Autodesk Inventor part; units mm, degrees
ref_plane "Work Plane1" through (0, 0, -15) normal (0, 0, 1) x (1, 0, 0)
ref_plane "YZ Plane" through (0, 0, 0) normal (1, 0, 0) x (0, 1, 0)
ref_plane "XZ Plane" through (0, 0, 0) normal (0, 1, 0) x (-1, 0, 0)
sketch "Sketch1" plane through (0, 0, 0) normal (0, 0, 1) x (1, 0, 0)
  line L0 (0, 0) -> (25, 0)
  line L1 (25, 0) -> (25, 40)
  line L2 (25, 40) -> (0, 40)
  line L3 (0, 40) -> (0, 0)
  dimension "d1" = 25
  dimension "d2" = 40
  dimension "d3" = 25
extrude "Extrusion1" add sketch "Sketch1" against normal blind 30
sketch "Sketch2" plane through (25, 0, 0) normal (1, 0, 0) x (0, 0, -1)
  line L0 (0, 0) -> (30, 0)
  circle A0 centre (15, 6.56) radius 2.46
extrude "Extrusion2" cut sketch "Sketch2" against normal blind 30
sketch "Sketch3" plane through (0, 0, 0) normal (-1, 0, 0) x (0, 0, 1)
  line L0 (0, 0) -> (-30, 0)
  line L1 (-25.05, 0) -> (-4.95, 0)
  line L2 (-4.95, 0) -> (-4.95, 33.12)
  line L3 (-4.95, 33.12) -> (-25.05, 33.12)
  line L4 (-25.05, 33.12) -> (-25.05, 0)
  dimension "d11" = 20.1
extrude "Extrusion3" cut sketch "Sketch3" against normal blind 20
sketch "Sketch4" plane through (0, 0, 0) normal (0, -1, 0) x (1, 0, 0)
  line L0 (20, -4.95) -> (20, -25.05)
  line L1 (20, -15) -> (25, -15)
  line L2 (25, 0) -> (25, -30)
  line L3 (20, -8.025) -> (25, -8.025)
  line L4 (25, -8.025) -> (25, -21.975)
  line L5 (25, -21.975) -> (20, -21.975)
  line L6 (20, -21.975) -> (20, -8.025)
  line L7 (20, -8.025) -> (25, -21.975) construction
  line L8 (25, -8.025) -> (20, -21.975) construction
  line L9 (25, -12.54) -> (25, -17.46)
  point P0 (0, 0)
  point P1 (22.5, -15)
  dimension "d14" = 13.95
extrude "Extrusion4" add sketch "Sketch4" along normal blind 15
sketch "Sketch5" plane through (20, 0, 0) normal (-1, 0, 0) x (0, 0, 1)
  circle A0 centre (-15, 6.56) radius 2.46
  circle A1 centre (-15, 6.56) radius 4.7025
  circle A2 centre (-15, 6.56) radius 2.46
  circle A3 centre (-15, 6.56) radius 2.46
  point P0 (0, 0)
  dimension "d17" = 9.405
extrude "Extrusion5" cut sketch "Sketch5" against normal blind 2.1
sketch "Sketch6" plane through (25, 0, 0) normal (1, 0, 0) x (0, 0, -1)
  circle A0 centre (15, 6.56) radius 4.7025
  line L0 (15, 6.56) -> (15, 23.56)
  circle A1 centre (15, 23.56) radius 2.46
  point P0 (0, 0)
  dimension "d20" = 17
  dimension "d21" = 4.92
extrude "Extrusion6" cut sketch "Sketch6" against normal blind 10 contours A1
sketch "Sketch7" plane through (20, 0, 0) normal (-1, 0, 0) x (0, 0, 1)
  circle A0 centre (-15, 23.56) radius 2.46
  circle A1 centre (-15, 23.56) radius 4.7025
  point P0 (0, 0)
  dimension "d24" = 9.405
extrude "Extrusion7" cut sketch "Sketch7" against normal blind 2.1
sketch "Sketch9" plane through (25, 0, 0) normal (1, 0, 0) x (0, 0, -1)
  circle A0 centre (15, 6.56) radius 2.46
  circle A1 centre (15, 6.56) radius 2.46
  circle A2 centre (15, 23.56) radius 2.46
  circle A3 centre (15, 23.56) radius 2.46
  line L0 (30, 40) -> (30, 0)
  line L1 (30, 0) -> (30, 40)
  line L2 (30, 40) -> (0, 40)
  line L3 (0, 40) -> (0, 0)
  line L4 (0, 0) -> (8.025, 0)
  line L5 (21.975, 0) -> (21.975, -15)
  line L6 (21.975, -15) -> (8.025, -15)
  line L7 (8.025, -15) -> (8.025, 0)
  line L8 (0, 0) -> (8.025, 0)
  line L9 (21.975, 0) -> (30, 0)
extrude "Extrusion8" add sketch "Sketch9" along normal blind 5
sketch "Sketch10" plane through (0, 40, 0) normal (0, 1, 0) x (1, 0, 0)
  line L0 (0, 30) -> (30, 30)
  line L1 (30, 0) -> (0, 0)
  line L2 (0, 30) -> (30, 30)
  line L3 (30, 30) -> (30, 0)
  line L4 (30, 0) -> (0, 0)
  line L5 (0, 0) -> (0, 30)
extrude "Extrusion9" add sketch "Sketch10" along normal blind 30
sketch "Sketch12" plane through (30, 0, 0) normal (1, 0, 0) x (0, 0, -1)
  circle A0 centre (15, 6.56) radius 2.46
  line L0 (15, 6.56) -> (15, 15.06)
  circle A1 centre (15, 15.06) radius 2.525
  point P0 (0, 0)
  dimension "d31" = 8.5
  dimension "d33" = 5.05
extrude "Extrusion10" cut sketch "Sketch12" against normal blind 30 contours A1
sketch "Sketch14" plane through (0, 0, 0) normal (0, 0, 1) x (1, 0, 0)
  line L0 (30, 70) -> (0, 70)
  line L1 (0, 100) -> (-8, 100)
  line L2 (30, 0) -> (30, 70)
  line L3 (30, 118) -> (30, 70)
  line L4 (30, 105) -> (30, 100)
  line L5 (0, 70) -> (30, 70)
  line L6 (0, 70) -> (0, 100)
  line L7 (-8, 145) -> (15, 145)
  line L8 (-2, 142.5) -> (-8, 145)
  line L9 (-2, 102.5) -> (-8, 100)
  line L10 (-2, 102.5) -> (4, 122.5)
  line L11 (4, 122.5) -> (-2, 142.5)
  line L12 (15, 145) -> (30, 122.5)
  line L13 (30, 122.5) -> (30, 118)
  point P0 (0, 0)
  dimension "d47" = 30
  dimension "d85" = 45
extrude "Extrusion12" add sketch "Sketch14" against normal blind 30
sketch "Sketch15" plane through (0, 0, -25.05) normal (-1, 0, 0) x (0, 0, 1)
  line L0 (0, 33.12) -> (20.1, 33.12)
  line L1 (20.1, 33.12) -> (20.1, 0)
  line L2 (0, 33.12) -> (20.1, 33.12)
  line L3 (20.1, 33.12) -> (20.1, 31.1)
  line L4 (20.1, 31.1) -> (0, 31.1)
  line L5 (0, 31.1) -> (0, 33.12)
  point P0 (25.05, 0)
  dimension "d57" = 2.02
extrude "Extrusion13" add sketch "Sketch15" against normal blind 20
sketch "Sketch25" plane through (0, 0, 0) normal (0, 0, 1) x (1, 0, 0)
  line L0 (-8, 100) -> (0, 100)
  line L1 (0, 100) -> (-8, 100)
  line L2 (-8, 100) -> (-2, 102.5)
  line L3 (-8, 100) -> (-2, 102.5)
  line L4 (-2, 102.5) -> (4, 122.5)
  line L5 (-8, 145) -> (-2, 142.5)
  line L6 (4, 122.5) -> (-2, 142.5)
  line L7 (-2, 142.5) -> (-8, 145)
  line L8 (15, 145) -> (-8, 145)
  line L9 (-8, 145) -> (15, 145)
  line L10 (15, 145) -> (30, 122.5)
  line L11 (15, 145) -> (30, 122.5)
  line L12 (30, 122.5) -> (30, 92.5)
  line L13 (30, 0) -> (30, 122.5)
  line L14 (30, 92.5) -> (0, 92.5)
  line L15 (0, 0) -> (0, 100)
  line L16 (0, 92.5) -> (0, 100)
  dimension "d88" = 30
extrude "Extrusion14" add sketch "Sketch25" along normal blind 15
ref_plane "Work Plane1" through (0, 0, -15) normal (0, 0, 1) x (1, 0, 0)
mirror "Mirror1" about plane through (0, 0, -15) normal (0, 0, 1) of "Extrusion14"
properties part number "40mm_x_60mm"
Can you work these out from the model? Positions are in its coordinate system, mm. A direction names the side the tool comes from. Coordinates: 2 decimals unless noted, no trailing zeros. Loops run counter-clockwise (first coordinate to the right, second up) from the corner with the lowest first, then second, coordinate; pieces in that order, holes last. Notation, with made-up numbers: M 86.25,-33.5 L 118.25,-33.5 A34 cw 118.25,-3.5 Z; hole C -32.75,17.5 d5. An arc over 180 degrees is marked long. Put each result on its own line as item: value. Start each with the question number.
(1) Imagine slicing it at A-A on y = 23.56. List the corners of the cut face in (x, z) for me, and give its area (3 significant figures).
(2) Imagine slicing it at C-C on z = 7.5. List the corners of the cut face in (x, y) for me, and give its area (3 significant figures).
(3) Imagine slicing it at B-B on x = 26.5. List the corners of the cut face in (y, z) for me (3 decimals), and give its area (3 significant figures).
(4) I need wall thicknesses on probe 1 along Y at (x, z) = (26, -15) (3 decimals); probe 2 along Y at (x, z) = (25, -15) (3 decimals); probe 3 along Z at (x, y) = (1, 72). Which ranges of each line are inside material? Lowest first, please.
(5) Which directions (+Z, -Z, +X, -X, +Y, -Y) give clear straight access to the entire face, cutting with the end or side of a thin tool? Please do faces 1 (the face through (22.1, 4.5, -13)), 2 (the face through (1.04, 112.64, -14.58)), 3 (the face through (10, 31.1, -15)).
(6) Will these pins go through, and if not, where does the flat tip stop? pin 1 Ø2 at (x, z) = (23.5, -26) entering from +Y; pin 2 Ø15 at (x, y) = (20, 54) entering from +Z; pin 3 Ø3 at (x, y) = (25, -5) entering from +Z (3 decimals).
(7) Imagine slicing it at D-D on x = 8. List the corners of the cut face in (y, z) for me, and give its area (3 significant figures).
(8) We'd pull the mould along Z, two halves only. Please class faces 4 (the face through (15, 47, -30)), 5 (the face through (10, 16, -25.05)), 6 (the face through (-4, 100, -15)), 7 (the face through (22.1, 21.5, -13)): +Z half, -Z half, draft (parallel to the pull), parting line (faces both ways), or undercut.
Worked answers:
1. outline: M 0,-30 L 30,-30 L 30,-17.46 L 22.1,-17.46 L 22.1,-19.7 L 20,-19.7 L 20,-25.05 L 0,-25.05 Z; M 0,-4.95 L 20,-4.95 L 20,-10.3 L 22.1,-10.3 L 22.1,-12.54 L 30,-12.54 L 30,0 L 0,0 Z
1. area: 439 mm2
2. outline: M -8,100 L 0,100 L 0,92.5 L 30,92.5 L 30,122.5 L 15,145 L -8,145 L -2,142.5 L 4,122.5 L -2,102.5 Z
2. area: 1,390 mm2
3. outline: M -15,-21.975 L 0,-21.975 L 0,-30 L 92.5,-30 L 92.5,-45 L 127.75,-45 L 127.75,15 L 92.5,15 L 92.5,0 L 0,0 L 0,-8.025 L -15,-8.025 Z; hole C 6.56,-15 d4.92; hole C 15.06,-15 d5.05; hole C 23.56,-15 d4.92
3. area: 5,040 mm2
4. probe 1: y = -15 to 4.1, 9.02 to 12.535, 17.585 to 21.1, 26.02 to 128.5
4. probe 2: y = -15 to 4.1, 9.02 to 12.535, 17.585 to 21.1, 26.02 to 130
4. probe 3: z = -30 to 0
5. face 1: -X
5. face 2: +Z, -Z, -X
5. face 3: -X, -Y
6. pin 1: stops at y = 133.75
6. pin 2: stops at z = 0
6. pin 3: stops at z = -8.025
7. outline: M 0,-30 L 92.5,-30 L 92.5,-45 L 145,-45 L 145,15 L 92.5,15 L 92.5,0 L 0,0 L 0,-4.95 L 31.1,-4.95 L 31.1,-25.05 L 0,-25.05 Z
7. area: 5,300 mm2
8. face 4: -Z half
8. face 5: undercut
8. face 6: draft
8. face 7: undercut
